Source: CAD feature listing. Evaluate the final solid. Frame: model axes, mm. A direction names the side the tool comes from. Coordinates: 2 decimals unless noted, no trailing zeros. Loops run counter-clockwise (first coordinate to the right, second up) from the corner with the lowest first, then second, coordinate; pieces in that order, holes last. Notation, with made-up numbers: (-22, 18) - (13, 18) arc R14 ccw to (13, 38) - close; hole circle Ø5 at (10, -2.75). An arc over 180 degrees is marked (long way). Use CSV: the item, a comma, the result in double quotes. Start each with the question number.
```python
from build123d import *

# Parameters (mm, degrees)
SKETCH1_R           = 10.5
SKETCH1_R_2         = 1.5
BOSS_EXTRUDE1_DEPTH = 2.5
SKETCH2_R           = 4.3
SKETCH2_R_2         = 2.7
BOSS_EXTRUDE2_DEPTH = 3
SKETCH3_R           = 0.75
CUT_EXTRUDE1_DEPTH  = 16.149257408
CIRPATTERN1_COUNT   = 4
SKETCH4_R           = 4.3
SKETCH4_R_2         = 2.7
SKETCH4_R_3         = 2.2
SKETCH4_R_4         = 1.5
CUT_EXTRUDE2_DEPTH  = 1


with BuildPart() as part:
    # Sketch1 → Boss-Extrude1 (new body)
    with BuildSketch(Plane(origin=(0, 0, 0), x_dir=(1, 0, 0), z_dir=(0, 1, 0))):
        with Locations(Location((0, 0, 0), (0, 0, 270))):
            Circle(SKETCH1_R)
        with Locations(Location((0, 0, 0), (0, 0, 270))):
            Circle(SKETCH1_R_2, mode=Mode.SUBTRACT)
    extrude(amount=BOSS_EXTRUDE1_DEPTH)

    # Sketch2 → Boss-Extrude2 (add)
    with BuildSketch(Plane(origin=(0, 2.5, 0), x_dir=(1, 0, 0), z_dir=(0, 1, 0))):
        with Locations(Location((0, 0, 0), (0, 0, 270))):
            Circle(SKETCH2_R)
        with Locations(Location((0, 0, 0), (0, 0, 270))):
            Circle(SKETCH2_R_2, mode=Mode.SUBTRACT)
    extrude(amount=BOSS_EXTRUDE2_DEPTH)

    # Sketch3 → Cut-Extrude1 (cut, through all)
    with BuildSketch(Plane(origin=(0, 2.5, 0), x_dir=(1, 0, 0), z_dir=(0, 1, 0))):
        with Locations(Location((0, 7, 0), (0, 0, 270))):
            Circle(SKETCH3_R)
        with Locations(Location((3.5, 7, 0), (0, 0, 270))):
            Circle(SKETCH3_R)
        with Locations(Location((-3.5, 7, 0), (0, 0, 270))):
            Circle(SKETCH3_R)
    cut_extrude1 = extrude(amount=-CUT_EXTRUDE1_DEPTH, mode=Mode.SUBTRACT)

    # CirPattern1: Cut-Extrude1 ×4 about axis
    cirpattern1_axis = Axis((0, 0, 0), (0, 1, 0))
    for i in range(1, CIRPATTERN1_COUNT):
        add(cut_extrude1.rotate(cirpattern1_axis, i * 360 / CIRPATTERN1_COUNT), mode=Mode.SUBTRACT)

    # Sketch4 → Cut-Extrude2 (cut)
    # profile 1 of 2: a face of its own
    with BuildSketch(Plane.XZ):
        with Locations(Location((0, 0, 0), (0, 0, 90))):
            Circle(SKETCH4_R)
        with Locations(Location((0, 0, 0), (0, 0, 90))):
            Circle(SKETCH4_R_2, mode=Mode.SUBTRACT)
    # profile 2 of 2: a face of its own
    with BuildSketch(Plane.XZ):
        with Locations(Location((0, 0, 0), (0, 0, 270))):
            Circle(SKETCH4_R_3)
        with Locations(Location((0, 0, 0), (0, 0, 270))):
            Circle(SKETCH4_R_4, mode=Mode.SUBTRACT)
    extrude(amount=-CUT_EXTRUDE2_DEPTH, mode=Mode.SUBTRACT)


solid = part.part
```
(1) Draft query along Z for faces 1 (the cylindrical face through (3.2, 1.2, 10)), 2 (the flat face through (0, 2.5, 5)), 3 (the cylindrical face through (7.75, 1.27, 0.03)). Return one class per face: released by +Z, released by -Z, zero draft, split by the parting line, or undercut.
(2) Ray query, line 1 (Z direction, x = -7, y = 0.8); line 2 (Y direction, x = 4.5, z = -7.75). Return the intervals inside material, ascending. Write a range as [from, to].
(3) Section B-B on z = -3.5. Output: boundary loops of the cut face in (x, y), plus the area to 3 significant figures.
(4) Section D-D on y = 3.2. Output: boundary loops of the cut face in (x, z).
(5) Section A-A on x = 6.75. Output: boundary loops of the cut face in (y, z), plus the area to 3 significant figures.
(6) Reachability of faces 4 (the cylindrical face through (-7.595, 1.268, 3.956)), 5 (the flat face through (-1.2, 2.5, 1.2)), 6 (the flat face through (-1.4, 1, -0.9)) from +Z, -Z, +X, -X, +Y, -Y: full face, straight path, thin tool, end or side. Return the list, or none.
(7) Section C-C on x = -3.75. Output: boundary loops of the cut face in (y, z), plus the area to 3 significant figures.
(8) Pin query (flat end, axial travel): pin 1 Ø3.5 at (x, z) = (0, 0) entering from -Y; pin 2 Ø1.7 at (x, z) = (-3.5, 7) entering from +Y; pin 3 Ø1 at (y, z) = (1, -7.5) entering from -X. Return the tip coordinate at first contact, or that it passes through.
Solution:
1,face 1,"split by the parting line"
1,face 2,"zero draft"
1,face 3,"undercut"
2,line 1,"z = [-7.83, -4.25], [-2.75, -0.75], [0.75, 2.75], [4.25, 7.83]"
2,line 2,"y = [0, 2.5]"
3,outline,"(-9.9, 0) - (-7.75, 0) - (-7.75, 2.5) - (-9.9, 2.5) - close; (-6.25, 0) - (-2.5, 0) - (-2.5, 1) - (2.5, 1) - (2.5, 0) - (6.25, 0) - (6.25, 2.5) - (2.5, 2.5) - (2.5, 5.5) - (-2.5, 5.5) - (-2.5, 2.5) - (-6.25, 2.5) - close; (7.75, 0) - (9.9, 0) - (9.9, 2.5) - (7.75, 2.5) - close"
3,area,"52.0 mm²"
4,outline,"circle Ø8.6 at (0, 0); hole circle Ø5.4 at (0, 0)"
5,outline,"(0, -8.04) - (2.5, -8.04) - (2.5, -4.21) - (0, -4.21) - close; (0, -2.79) - (2.5, -2.79) - (2.5, -0.71) - (0, -0.71) - close; (0, 0.71) - (2.5, 0.71) - (2.5, 2.79) - (0, 2.79) - close; (0, 4.21) - (2.5, 4.21) - (2.5, 8.04) - (0, 8.04) - close"
5,area,"29.6 mm²"
6,face 4,"+Y, -Y"
6,face 5,"+Y"
6,face 6,"-Y"
7,outline,"(0, -9.81) - (2.5, -9.81) - (2.5, -7.71) - (0, -7.71) - close; (0, -6.29) - (2.5, -6.29) - (2.5, -2.1) - (5.5, -2.1) - (5.5, 2.1) - (2.5, 2.1) - (2.5, 6.29) - (0, 6.29) - (0, 2.1) - (1, 2.1) - (1, -2.1) - (0, -2.1) - close; (0, 7.71) - (2.5, 7.71) - (2.5, 9.81) - (0, 9.81) - close"
7,area,"50.4 mm²"
8,pin 1,"stops at y = 1"
8,pin 2,"stops at y = 2.5"
8,pin 3,"stops at x = -7.83"
